from build123d import *

# Parameters (mm, degrees)
SKETCH1_W               = 101.6
SKETCH1_H               = 50.8
BOSS_EXTRUDE1_DEPTH     = 101.6
CUT_EXTRUDE1_DEPTH      = 153.4
CUT_EXTRUDE1_DEPTH_BACK = 153.4
CUT_EXTRUDE2_DEPTH      = 153.4
CUT_EXTRUDE2_DEPTH_BACK = 153.4
SKETCH3_W               = 12.7
SKETCH3_H               = 50.8


with BuildPart() as part:
    # Sketch1 → Boss-Extrude1 (new body)
    with BuildSketch(Plane(origin=(0, 0, 0), x_dir=(1, 0, 0), z_dir=(0, 1, 0))):
        with Locations((-50.8, 25.4)):
            Rectangle(SKETCH1_W, SKETCH1_H)
    extrude(amount=BOSS_EXTRUDE1_DEPTH)

    # Sketch2 → Cut-Extrude1 (cut, two sides: drawn at the far end of the back side and taken through both)
    with BuildSketch(Plane(origin=(0, 101.6, 0), x_dir=(1, 0, 0), z_dir=(0, 1, 0)).offset(-CUT_EXTRUDE1_DEPTH_BACK)):
        Polygon((85.31205923, -122.77705923), (-37.465, 0), (-47.792294539, 10.327294539), (-58.119589078, 0), (-180.896648308, -122.77705923), (-180.896648308, -470.043023852), (85.31205923, -470.043023852), align=None)
    extrude(amount=CUT_EXTRUDE1_DEPTH + CUT_EXTRUDE1_DEPTH_BACK, mode=Mode.SUBTRACT)

    # Sketch3 → Cut-Extrude2 (cut, two sides: drawn at the far end of the back side and taken through both)
    with BuildSketch(Plane.XZ.offset(-CUT_EXTRUDE2_DEPTH_BACK)):
        with Locations((-95.25, -25.4)):
            Rectangle(SKETCH3_W, SKETCH3_H)
    extrude(amount=CUT_EXTRUDE2_DEPTH + CUT_EXTRUDE2_DEPTH_BACK, mode=Mode.SUBTRACT)


solid = part.part
Geometry check sheet. Reference: the model listing, model coordinates, mm. A direction names the side the tool comes from. Round coordinates to 2 decimals unless told otherwise and drop trailing zeros. Write each loop counter-clockwise with the first axis right and the second up, starting at its lowest first coordinate (ties: lowest second). Pieces come first, ordered by that corner, then holes.
Item 1: Section check B-B (z = -6.5). Record the boundary of the cut face in (x, y) (3 decimals), plus the area to 3 significant figures.
Determined:
outline: (-88.9, 0) - (-51.62, 0) - (-51.62, 101.6) - (-88.9, 101.6) - close; (-43.965, 0) - (0, 0) - (0, 101.6) - (-43.965, 101.6) - close
area: 8,250 mm2
Item 2: Section check A-A (y = 60). Record the boundary of the cut face in (x, z) (3 decimals), plus the area to 3 significant figures.
Determined:
outline: (-88.9, -50.8) - (0, -50.8) - (0, 0) - (-37.465, 0) - (-47.792, -10.327) - (-58.12, 0) - (-88.9, 0) - close
area: 4,410 mm2
Item 3: Access from +Z, -Z, +X, -X, +Y, -Y to the whole of each face (thin tool, end or side, straight path). Record for faces 5 (the face through (-45, 50, -50.8)), 6 (the face through (-42.556, 50.089, -5.091)).
Determined:
face 5: -Z, +X, -X, +Y, -Y
face 6: +Z, +Y, -Y
Item 4: Mould release check, pull along X, two halves, no side actions. Record for faces 1 (the face through (-52.88, 50.09, -5.24)), 2 (the face through (0, 50, -25)), 3 (the face through (-45, 101.6, -26)), 4 (the face through (-88.9, 52, -26)): +X half, -X half, draft (parallel to the pull), parting line (faces both ways), or undercut.
Determined:
face 1: undercut
face 2: +X half
face 3: draft
face 4: -X half
Item 5: Section check C-C (x = -53). Record the boundary of the cut face in (y, z).
Determined:
outline: (0, -50.8) - (101.6, -50.8) - (101.6, -5.12) - (0, -5.12) - close
Item 6: Material ranges on line 1 along X through (y, z) = (4, -6) (3 decimals); line 2 along X through (y, z) = (84.5, -7.5) (3 decimals); line 3 along Z through (x, y) = (-54.5, 17.5), recorded low to high.
Determined:
line 1: x = -88.9 to -52.12, -43.465 to 0
line 2: x = -88.9 to -50.62, -44.965 to 0
line 3: z = -50.8 to -3.62
